from build123d import *

# Parameters (mm, degrees)
F0_W     = 25.4
F0_H     = 9
F1_DEPTH = 3
F2_W     = 6.3
F2_H     = 9
F3_DEPTH = 9
F5_DEPTH = 25
F6_DEPTH = 25
F8_D     = 5.1054
F9_D     = 3.2


with BuildPart() as f1:
    # F0 (on Top) → F1 (new body)
    with BuildSketch(Plane.XY):
        Rectangle(F0_W, F0_H)
    extrude(amount=F1_DEPTH)

    # F2 (on face) → F3 (join)
    with BuildSketch(Plane.XY.offset(3)):
        with Locations((-9.55, 0)):
            Rectangle(F2_W, F2_H)
        with Locations((9.55, 0)):
            Rectangle(F2_W, F2_H)
    extrude(amount=F3_DEPTH)

    # F4 (on face) → F5 (cut)
    with BuildSketch(Plane.YZ.offset(12.7)):
        with BuildLine():
            ThreePointArc((-4.5, 8.2006715238), (-0.0114142109, 11.9599530691), (4.5, 8.2280980423))
            Line((4.5, 8.2280980423), (4.5, 12))
            Line((4.5, 12), (-4.5, 12))
            Line((-4.5, 12), (-4.5, 8.2006715238))
        make_face()
    extrude(amount=-F5_DEPTH, mode=Mode.SUBTRACT)

    # F6 (cut): a face of the model
    f6_faces = [f1.faces().sort_by_distance(p)[0] for p in [
        (-12.3, -0.0114439809, 11.9697221024),
    ]]
    extrude(f6_faces, amount=-F6_DEPTH, mode=Mode.SUBTRACT)

    # F8 (through all)
    with Locations(Plane(origin=(-12.7, 0, 0), x_dir=(0, -1, 0), z_dir=(-1, 0, 0))):
        with Locations((0, 8.1223854795)):
            Hole(F8_D / 2)

    # F9 (through all)
    with Locations(Plane(origin=(0, 0, 0), x_dir=(1, 0, 0), z_dir=(0, 0, -1))):
        with Locations((0, 0)):
            Hole(F9_D / 2)


solid = f1.part
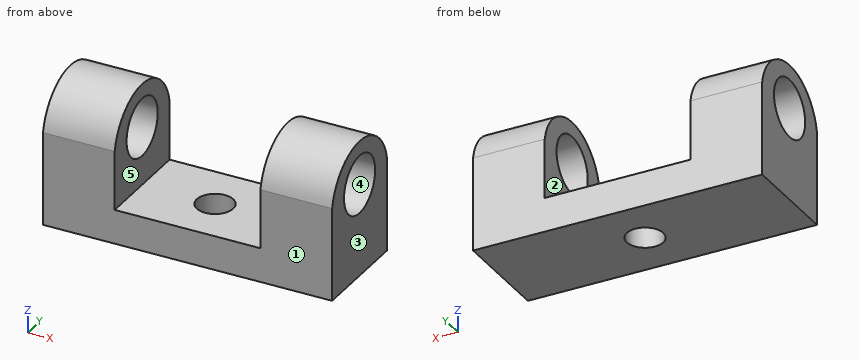
For this review, take the finished solid that the model builds, in its own axes (mm). Face numbers are marked on the shaded views. A direction names the side the tool comes from. Give positions to 0.01 mm unless a question says otherwise; leave off trailing zeros. Loops run counter-clockwise (first coordinate to the right, second up) from the corner with the lowest first, then second, coordinate; pieces in that order, holes last. Notation, with made-up numbers: M -38.5,-14 L -23.5,-14 A31 cw -23.5,16 Z; hole C 26.25,23.25 d5. An arc over 180 degrees is marked long. Answer as a JSON object with one key per item and string values. Group by question number.
Q1. Add section B-B on z = 5. Give the boundary of the cut face in (x, y), and give its area (3 significant figures).
Q2. Add section C-C on y = 0. Give the boundary of the cut face in (x, z).
Q3. Mouldability with a two-part tool opening along X and no side actions: class the marked faces 1, 2 and 3 as +X half, -X half, draft (parallel to the pull), parting line (faces both ways), or undercut.
Q4. Add section A-A on x = 0. Give the boundary of the cut face in (y, z).
Q5. Insertion check: P1, Ø2, axis at y = 2, z = 7, coming from the +X side. The pin has a flat end and moves straight along its axis. Give the tip position at first contact, or say it passes through.
Q6. For probe 1 along X at (y, z) = (4, 8); probe 2 along Z at (x, y) = (8.5, 0); probe 3 along Y at (x, z) = (0, 0.7), list the stretches that pass through material, from the lowest coordinate up. Write a range as [from, to].
Q7. Tool access review of the marked faces 4 and 5: name each direction out of +Z, -Z, +X, -X, +Y, -Y from which nothing blocks a thin tool from reaching the whole face with its end or side.
Q8. Add section D-D on z = 8.5. Give the boundary of the cut face in (x, y), and give its area (3 significant figures).
Checked values:
{
 "1": {"outline": "M -12.7,-4.5 L -6.4,-4.5 L -6.4,4.5 L -12.7,4.5 Z; M 6.4,-4.5 L 12.7,-4.5 L 12.7,4.5 L 6.4,4.5 Z", "area": "113 mm²"},
 "2": {"outline": "M -12.7,0 L -1.6,0 L -1.6,3 L -6.4,3 L -6.4,5.57 L -12.7,5.57 Z; M -12.7,10.68 L -6.4,10.68 L -6.4,11.96 L -12.7,11.96 Z; M 1.6,0 L 12.7,0 L 12.7,5.57 L 6.4,5.57 L 6.4,3 L 1.6,3 Z; M 6.4,10.68 L 12.7,10.68 L 12.7,11.96 L 6.4,11.96 Z"},
 "3": {"face 1": "draft", "face 2": "undercut", "face 3": "+X half"},
 "4": {"outline": "M -4.5,0 L -1.6,0 L -1.6,3 L -4.5,3 Z; M 1.6,0 L 4.5,0 L 4.5,3 L 1.6,3 Z"},
 "5": {"P1": "x = 12.7"},
 "6": {"probe 1": "[-12.7, -6.4], [6.4, 12.7]", "probe 2": "[0, 5.57], [10.68, 11.96]", "probe 3": "[-4.5, -1.6], [1.6, 4.5]"},
 "7": {"face 4": "+X, -X", "face 5": "+Z, +Y, -Y"},
 "8": {"outline": "M -12.7,-4.44 L -6.4,-4.44 L -6.4,-2.52 L -12.7,-2.52 Z; M -12.7,2.52 L -6.4,2.52 L -6.4,4.44 L -12.7,4.44 Z; M 6.4,-4.44 L 12.7,-4.44 L 12.7,-2.52 L 6.4,-2.52 Z; M 6.4,2.52 L 12.7,2.52 L 12.7,4.44 L 6.4,4.44 Z", "area": "48.2 mm²"}
}
